Could you check a few things on this model? Use its own coordinates, in mm. A direction names the side the tool comes from. Give positions to 0.01 mm unless a question says otherwise; leave off trailing zeros. Write each loop counter-clockwise with the first axis right and the second up, starting at its lowest first coordinate (ties: lowest second). Pieces come first, ordered by that corner, then holes. Notation, with made-up numbers: M 58.25,20 L 99.25,20 A11 ccw 99.25,26 Z; hole C 7.5,38 d6. An arc over 180 degrees is marked long. One line per item, written item: value.
```python
from build123d import *

# Parameters (mm, degrees)
BOSS_EXTRUDE1_DEPTH                  = 2.5
F_6_2_6_2_DIAMETER_HOLE1_D           = 6.2
F_6_2_6_2_DIAMETER_HOLE1_CSINK_D     = 6.25
F_6_2_6_2_DIAMETER_HOLE1_CSINK_ANGLE = 90


with BuildPart() as part:
    # Sketch1 → Boss-Extrude1 (new, symmetric)
    with BuildSketch(Plane(origin=(0, 0, 0), x_dir=(1, 0, 0), z_dir=(0, 1, 0))):
        Polygon((45, 15), (35, 15), (35, 10), (25, 10), (25, 15), (15, 15), (15, 10), (5, 10), (5, 15), (-5, 15), (-5, 10), (-15, 10), (-15, 15), (-25, 15), (-25, 10), (-35, 10), (-35, 15), (-45, 15), (-45, 10), (-55, 10), (-55, 5), (-60, 5), (-60, -5), (-55, -5), (-55, -10), (-45, -10), (-45, -15), (-35, -15), (-35, -10), (-25, -10), (-25, -15), (-15, -15), (-15, -10), (-5, -10), (-5, -15), (5, -15), (5, -10), (15, -10), (15, -15), (25, -15), (25, -10), (35, -10), (35, -15), (45, -15), (45, -10), (55, -10), (55, -5), (60, -5), (60, 5), (55, 5), (55, 10), (45, 10), align=None)
    extrude(amount=BOSS_EXTRUDE1_DEPTH, both=True)

    # Ø6.2 (6.2) Diameter Hole1 (through all)
    with Locations(Plane(origin=(0, 2.5, 0), x_dir=(1, 0, 0), z_dir=(0, 1, 0))):
        with Locations((-45, 4.5), (45, 4.5)):
            CounterSinkHole(F_6_2_6_2_DIAMETER_HOLE1_D / 2, F_6_2_6_2_DIAMETER_HOLE1_CSINK_D / 2, counter_sink_angle=F_6_2_6_2_DIAMETER_HOLE1_CSINK_ANGLE)


solid = part.part
```
1) Please list where these lines run through material, in increasing order: L1, parallel to X at y = -1.05, z = 10.5; L2, parallel to Z at x = -53, y = 1.25; L3, parallel to X at y = 0.7, z = -6.25. Write a range as from..to.
Outcome:
L1: x = -45..-35, -25..-15, -5..5, 15..25, 35..45
L2: z = -10..10
L3: x = -55..-47.56, -42.44..42.44, 47.56..55
2) I'm going to push flat-ended pins straight in: pin 1 (2.5 mm diameter, centred on y = -1, z = 12, fed in from +X); pin 2 (3 mm diameter, centred on y = 0, z = 8.5, fed in from +X); pin 3 (2.5 mm diameter, centred on y = 1, z = -13, fed in from -X). Where does each tip first touch, or does it pass through?
Outcome:
pin 1: stops at x = 45
pin 2: stops at x = 55
pin 3: stops at x = -45
3) If we section it at B-B, the plane y = 1.7: Give the number of separate pieces and of enclosed holes in the cut face, then the cut area to 3 significant figures.
Outcome:
separate pieces: 1
enclosed holes: 2
area: 2,740 mm^2
4) If we section it at A-A, the plane z = -11.5: Write out the boundary of the cut face in (x, y), then the cut area to 3 significant figures.
Outcome:
outline: M -45,-2.5 L -35,-2.5 L -35,2.5 L -45,2.5 Z; M -25,-2.5 L -15,-2.5 L -15,2.5 L -25,2.5 Z; M -5,-2.5 L 5,-2.5 L 5,2.5 L -5,2.5 Z; M 15,-2.5 L 25,-2.5 L 25,2.5 L 15,2.5 Z; M 35,-2.5 L 45,-2.5 L 45,2.5 L 35,2.5 Z
area: 250 mm^2
5) We'd pull the mould along X, two halves only. Please class faces 6 (the face through (5, 0, 13)), 7 (the face through (60, 0, 0)), 8 (the face through (-57, 0, -5)): pulls with the +X half, pulls with the -X half, needs draft (parallel to the pull), parting line crosses it, or undercut.
Outcome:
face 6: undercut
face 7: pulls with the +X half
face 8: needs draft
6) On a 3-axis mill with a long thin cutter (end or side, diameter ignored), from which of +Z, -Z, +X, -X, +Y, -Y can I reach the whole of each face in a straight line? I mean faces 1 (the face through (-55, 0, -8)), 2 (the face through (45, 0, -12)), 3 (the face through (-30, 0, 10)), 4 (the face through (55, 0, 8)), 5 (the face through (-30, 0, -10)). Say none if no direction works.
Outcome:
face 1: -Z, -X, +Y, -Y
face 2: -Z, +X, +Y, -Y
face 3: +Z, +Y, -Y
face 4: +Z, +X, +Y, -Y
face 5: -Z, +Y, -Y
